from build123d import *

# Parameters (mm, degrees)
SKETCH1_R           = 5
BOSS_EXTRUDE1_DEPTH = 36
SKETCH2_R           = 6
BOSS_EXTRUDE2_DEPTH = 150
CHAMFER1_SIZE       = 1


with BuildPart() as part:
    # Sketch1 → Boss-Extrude1 (new body)
    with BuildSketch(Plane.XY):
        Circle(SKETCH1_R)
    extrude(amount=BOSS_EXTRUDE1_DEPTH)

    # Sketch2 → Boss-Extrude2 (add)
    with BuildSketch(Plane.XY.offset(36)):
        Circle(SKETCH2_R)
    extrude(amount=BOSS_EXTRUDE2_DEPTH)

    # Chamfer1
    chamfer1_edges = [part.edges().sort_by_distance(p)[0] for p in [
        (-5, 0, 0),
        (-6, 0, 186),
    ]]
    chamfer(chamfer1_edges, length=CHAMFER1_SIZE)


solid = part.part
CAD build for the part. Positions are in the model's coordinates, mm. A direction names the side the tool comes from. Coordinates: 2 decimals unless noted, no trailing zeros. Loops run counter-clockwise (first coordinate to the right, second up) from the corner with the lowest first, then second, coordinate; pieces in that order, holes last. Notation, with made-up numbers: (35.5, 3) - (82.5, 3) arc R28 ccw to (82.5, 26) - close; hole circle Ø1 at (66, -7.5). An arc over 180 degrees is marked (long way). Use one line per item in the form item = value. Start each with the question number.
1) Tool access for faces 1 (the face through (0, 0, 0)), 2 (the face through (-4, 4, 36)): list every direction of +Z, -Z, +X, -X, +Y, -Y with a clear straight run to the whole face (end or side of a thin tool).
2) Drill centre lines: L1, parallel to Y at x = 0.5, z = 39; L2, parallel to X at y = -1.5, z = 122.5; L3, parallel to Z at x = -2, y = 3.5. Where is each one in solid material? Low to high. Write a range as from..to.
3) Band-saw the part on C-C (z = 33.5). Give the cut face in (x, y).
4) Flat gauge pins, fed straight in: pin 1 (1 mm diameter, centred on x = 4, z = 113.5, fed in from +Y); pin 2 (1.5 mm diameter, centred on x = -2.5, z = 36.5, fed in from +Y); pin 3 (4 mm diameter, centred on y = -3.5, z = 44.5, fed in from -X). Where does each tip first touch, or does it go through?
5) Band-saw the part on A-A (y = 0). Give the cut face in (x, z), and give its area (3 significant figures).
6) Band-saw the part on D-D (z = 67.5). Give the cut face in (x, y), and give its area (3 significant figures).
Check values:
q1.face_1 = -Z, +X, -X, +Y, -Y
q1.face_2 = -Z
q2.L1 = -5.98..5.98
q2.L2 = -5.81..5.81
q2.L3 = 0.03..186
q3.outline = circle Ø10 at (0, 0)
q4.pin_1 = 4.87
q4.pin_2 = 5.74
q4.pin_3 = -5.81
q5.outline = (-6, 36) - (-5, 36) - (-5, 1) - (-4, 0) - (4, 0) - (5, 1) - (5, 36) - (6, 36) - (6, 185) - (5, 186) - (-5, 186) - (-6, 185) - close
q5.area = 2,160 mm2
q6.outline = circle Ø12 at (0, 0)
q6.area = 113 mm2
